For this review, take the finished solid that the model builds, in its own axes (mm). A direction names the side the tool comes from. Give positions to 0.01 mm unless a question says otherwise; leave off trailing zeros. Loops run counter-clockwise (first coordinate to the right, second up) from the corner with the lowest first, then second, coordinate; pieces in that order, holes last.
```python
from build123d import *

# Parameters (mm, degrees)
F1_DEPTH = 150
F2_R     = 11
F3_DEPTH = 38.101
F4_R     = 11
F5_DEPTH = 38.101


with BuildPart() as f1:
    # F0 (on Right) → F1 (new body)
    with BuildSketch(Plane.YZ):
        Polygon((0, 38.1), (0, 0), (1.5875, 0), (1.5875, 36.5125), (38.1, 36.5125), (38.1, 38.1), align=None)
    extrude(amount=F1_DEPTH)

    # F2 (on face) → F3 (cut, through all)
    with BuildSketch(Plane.XZ):
        with Locations((75, 19.05)):
            Circle(F2_R)
        with Locations((103, 19.05)):
            Circle(F2_R)
        with Locations((131, 19.05)):
            Circle(F2_R)
        with Locations((47, 19.05)):
            Circle(F2_R)
        with Locations((19, 19.05)):
            Circle(F2_R)
        with BuildLine():
            ThreePointArc((87, 0), (83, 4), (79, 0))
            Line((79, 0), (87, 0))
        make_face()
        with BuildLine():
            Line((91, 0), (99, 0))
            ThreePointArc((99, 0), (95, 4), (91, 0))
        make_face()
        with BuildLine():
            Line((103, 0), (111, 0))
            ThreePointArc((111, 0), (107, 4), (103, 0))
        make_face()
        with BuildLine():
            Line((115, 0), (123, 0))
            ThreePointArc((123, 0), (119, 4), (115, 0))
        make_face()
        with BuildLine():
            Line((127, 0), (135, 0))
            ThreePointArc((135, 0), (131, 4), (127, 0))
        make_face()
        with BuildLine():
            Line((139, 0), (147, 0))
            ThreePointArc((147, 0), (143, 4), (139, 0))
        make_face()
        with BuildLine():
            ThreePointArc((71, 0), (67, 4), (63, 0))
            Line((63, 0), (71, 0))
        make_face()
        with BuildLine():
            ThreePointArc((11, 0), (7, 4), (3, 0))
            Line((3, 0), (11, 0))
        make_face()
        with BuildLine():
            ThreePointArc((35, 0), (31, 4), (27, 0))
            Line((27, 0), (35, 0))
        make_face()
        with BuildLine():
            ThreePointArc((23, 0), (19, 4), (15, 0))
            Line((15, 0), (23, 0))
        make_face()
        with BuildLine():
            Line((39, 0), (47, 0))
            ThreePointArc((47, 0), (43, 4), (39, 0))
        make_face()
        with BuildLine():
            Line((51, 0), (59, 0))
            ThreePointArc((59, 0), (55, 4), (51, 0))
        make_face()
    extrude(amount=-F3_DEPTH, mode=Mode.SUBTRACT)

    # F4 (on face) → F5 (cut, through all)
    with BuildSketch(Plane.XY.offset(38.1)):
        with Locations((75, 19.05)):
            Circle(F4_R)
        with Locations((47, 19.05)):
            Circle(F4_R)
        with Locations((19, 19.05)):
            Circle(F4_R)
        with Locations((103, 19.05)):
            Circle(F4_R)
        with Locations((131, 19.05)):
            Circle(F4_R)
        with BuildLine():
            ThreePointArc((64.900003, 41.50441), (67, 34.1), (69.099998, 41.50441))
            Line((69.099998, 41.50441), (64.900003, 41.50441))
        make_face()
        with BuildLine():
            Line((57.099998, 41.50441), (52.900003, 41.50441))
            ThreePointArc((52.900003, 41.50441), (55, 34.1), (57.099998, 41.50441))
        make_face()
        with BuildLine():
            Line((45.099998, 41.50441), (40.900003, 41.50441))
            ThreePointArc((40.900003, 41.50441), (43, 34.1), (45.099998, 41.50441))
        make_face()
        with BuildLine():
            Line((33.099998, 41.50441), (28.900003, 41.50441))
            ThreePointArc((28.900003, 41.50441), (31, 34.1), (33.099998, 41.50441))
        make_face()
        with BuildLine():
            Line((21.099998, 41.50441), (16.900003, 41.50441))
            ThreePointArc((16.900003, 41.50441), (19, 34.1), (21.099998, 41.50441))
        make_face()
        with BuildLine():
            Line((9.099998, 41.50441), (4.900003, 41.50441))
            ThreePointArc((4.900003, 41.50441), (7, 34.1), (9.099998, 41.50441))
        make_face()
        with BuildLine():
            ThreePointArc((80.900003, 41.50441), (83, 34.1), (85.099998, 41.50441))
            Line((85.099998, 41.50441), (80.900003, 41.50441))
        make_face()
        with BuildLine():
            ThreePointArc((140.900003, 41.50441), (143, 34.1), (145.099998, 41.50441))
            Line((145.099998, 41.50441), (140.900003, 41.50441))
        make_face()
        with BuildLine():
            ThreePointArc((116.900003, 41.50441), (119, 34.1), (121.099998, 41.50441))
            Line((121.099998, 41.50441), (116.900003, 41.50441))
        make_face()
        with BuildLine():
            ThreePointArc((128.900003, 41.50441), (131, 34.1), (133.099998, 41.50441))
            Line((133.099998, 41.50441), (128.900003, 41.50441))
        make_face()
        with BuildLine():
            Line((109.099998, 41.50441), (104.900003, 41.50441))
            ThreePointArc((104.900003, 41.50441), (107, 34.1), (109.099998, 41.50441))
        make_face()
        with BuildLine():
            Line((97.099998, 41.50441), (92.900003, 41.50441))
            ThreePointArc((92.900003, 41.50441), (95, 34.1), (97.099998, 41.50441))
        make_face()
    extrude(amount=-F5_DEPTH, mode=Mode.SUBTRACT)


solid = f1.part
```
Q1. Consider section A-A on x = 75. Give the boundary of the cut face in (y, z).
Answers:
outline: (0, 0) - (1.59, 0) - (1.59, 8.05) - (0, 8.05) - close; (0, 30.05) - (1.59, 30.05) - (1.59, 36.51) - (8.05, 36.51) - (8.05, 38.1) - (0, 38.1) - close; (30.05, 36.51) - (38.1, 36.51) - (38.1, 38.1) - (30.05, 38.1) - close
Q2. Consider section B-B on z = 20.5. Give the boundary of the cut face in (x, y).
Answers:
outline: (0, 0) - (8.1, 0) - (8.1, 1.59) - (0, 1.59) - close; (29.9, 0) - (36.1, 0) - (36.1, 1.59) - (29.9, 1.59) - close; (57.9, 0) - (64.1, 0) - (64.1, 1.59) - (57.9, 1.59) - close; (85.9, 0) - (92.1, 0) - (92.1, 1.59) - (85.9, 1.59) - close; (113.9, 0) - (120.1, 0) - (120.1, 1.59) - (113.9, 1.59) - close; (141.9, 0) - (150, 0) - (150, 1.59) - (141.9, 1.59) - close
Q3. Machinability: for faces 5 (the cylindrical face through (30.9, 34.1, 37.3)), 6 (the flat face through (74, 1.588, 30.2)), which of the approach directions +Z, -Z, +X, -X, +Y, -Y give a long, thin tool a straight path to every point of the face, cutting with its end or side? Answer none if there is none.
Answers:
face 5: +Z, -Z, +Y
face 6: -Z, +X, -X, +Y
Q4. Mouldability with a two-part tool opening along Y and no side actions: class faces 1 (the cylindrical face through (19, 1, 4)), 2 (the cylindrical face through (120.01, 19.53, 37.32)), 3 (the cylindrical face through (118.9, 34.1, 37.3)), 4 (the flat face through (74, 0, 32)) as +Y half, -Y half, draft (parallel to the pull), parting line (faces both ways), or undercut.
Answers:
face 1: draft
face 2: undercut
face 3: +Y half
face 4: -Y half
Q5. For probe 1 along Y at (x, z) = (131, 37.7); probe 2 along Z at (x, y) = (38, 30); probe 3 along Y at (x, z) = (64, 34.5), list the stretches that pass through material, from the lowest coordinate up.
Answers:
probe 1: y = 0 to 8.05, 30.05 to 34.1
probe 2: z = 36.51 to 38.1
probe 3: y = 0 to 1.59
Q6. Consider section C-C on y = 27. Give the boundary of the cut face in (x, z), plus the area to 3 significant figures.
Answers:
outline: (0, 36.51) - (11.4, 36.51) - (11.4, 38.1) - (0, 38.1) - close; (26.6, 36.51) - (39.4, 36.51) - (39.4, 38.1) - (26.6, 38.1) - close; (54.6, 36.51) - (67.4, 36.51) - (67.4, 38.1) - (54.6, 38.1) - close; (82.6, 36.51) - (95.4, 36.51) - (95.4, 38.1) - (82.6, 38.1) - close; (110.6, 36.51) - (123.4, 36.51) - (123.4, 38.1) - (110.6, 38.1) - close; (138.6, 36.51) - (150, 36.51) - (150, 38.1) - (138.6, 38.1) - close
area: 117 mm2
Q7. Consider section D-D on y = 6.5. Give the boundary of the cut face in (x, z).
Answers:
outline: (0, 36.51) - (150, 36.51) - (150, 38.1) - (0, 38.1) - close
Q8. For pin 1 Ø18.5 at (x, y) = (74, 12) entering from -Z; pin 2 Ø20 at (x, z) = (19, 19.05) entering from +Y; pin 3 Ø4 at (x, z) = (49.5, 5.5) entering from +Y, all flat-tipped, find the tip position at first contact; note any pin that passes through.
Answers:
pin 1: stops at z = 36.51
pin 2: passes through
pin 3: stops at y = 1.59
